Answer from the drawing. Dimensions are ordinates in mm from the lowest x, y and z of the part. A direction names the side the tool comes from. Coordinates: 2 decimals unless noted, no trailing zeros. Write each loop counter-clockwise with the first axis right and the second up, starting at its lowest first coordinate (ties: lowest second). Pieces come first, ordered by that corner, then holes. Notation, with made-up numbers: (26.25, 22) -> (41.25, 22) arc R32 cw to (41.25, 48) -> close; hole circle Ø2 at (56, 65). An arc over 180 degrees is marked (long way). Return JSON: item names as keys, results as strings.
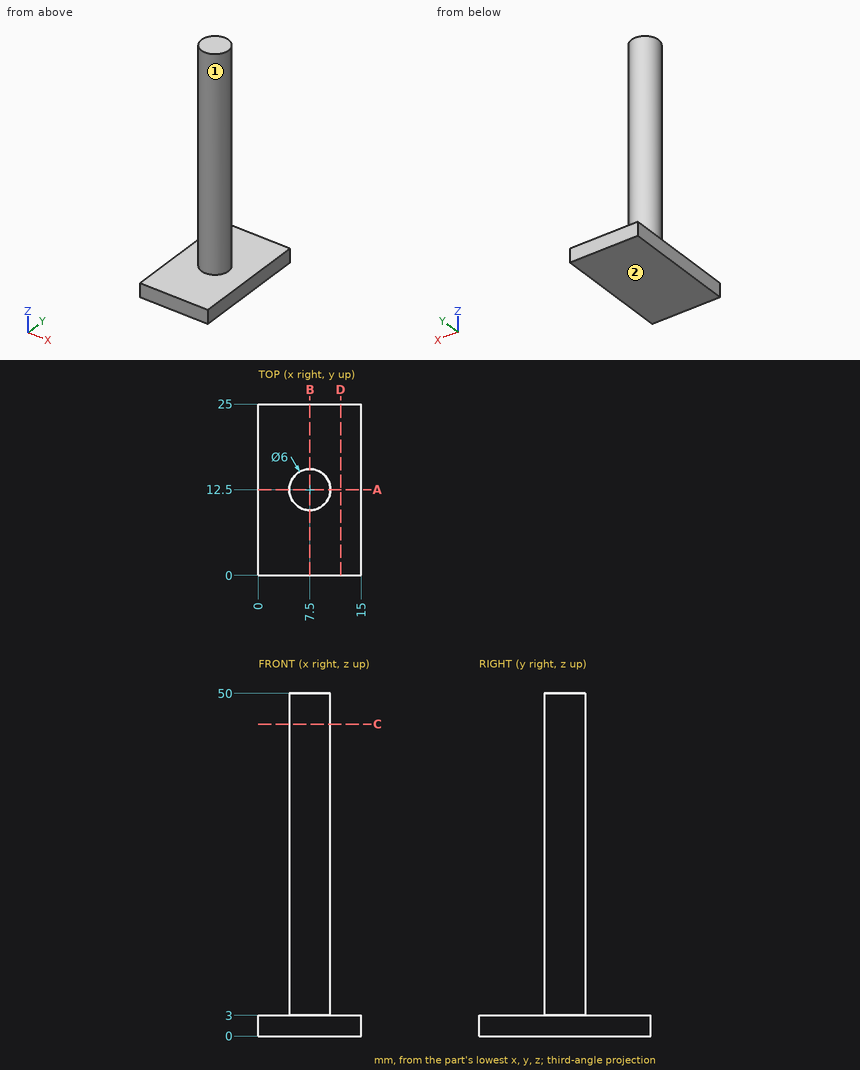
1. The part is cut by section D-D (x = 12). Determine the outline of the cut face in (y, z), then the cut area to 3 significant figures.
Taken from the geometry:
{"outline": "(0, 0) -> (25, 0) -> (25, 3) -> (0, 3) -> close", "area": "75.0 mm2"}
2. Flat-ended cylindrical pins translate along their axes: pin 1 Ø10 at (y, z) = (21, 36.5) entering from +X; pin 2 Ø7.5 at (x, y) = (7.5, 16.5) entering from +Z; pin 3 Ø6 at (x, z) = (4.5, 12) entering from -Y; pin 4 Ø1 at (x, z) = (10, 43) entering from -Y. Find the tip coordinate at first contact, or state that the pin passes through.
Taken from the geometry:
{"pin 1": "passes through", "pin 2": "stops at z = 50", "pin 3": "stops at y = 9.5", "pin 4": "stops at y = 10.26"}
3. The part is cut by section B-B (x = 7.5). Determine the outline of the cut face in (y, z).
Taken from the geometry:
{"outline": "(0, 0) -> (25, 0) -> (25, 3) -> (15.5, 3) -> (15.5, 50) -> (9.5, 50) -> (9.5, 3) -> (0, 3) -> close"}
4. A tool of negligible diameter and unlimited length cuts with its end or side. For the marked faces 1 and 2, from which of +Z, -Z, +X, -X, +Y, -Y can it reach the whole face along a straight path? Write none if from no direction.
Taken from the geometry:
{"face 1": "+Z", "face 2": "-Z, +X, -X, +Y, -Y"}
5. Consider L1, parallel to Z at x = 1.25, y = 14.75; L2, parallel to X at y = 12.5, z = 21.5; L3, parallel to X at y = 10.5, z = 21. Determine where each line is inside the solid, lowest interval first.
Taken from the geometry:
{"L1": "z = 0 to 3", "L2": "x = 4.5 to 10.5", "L3": "x = 5.26 to 9.74"}
6. The part is cut by section C-C (z = 45.5). Determine the outline of the cut face in (x, y), then the cut area to 3 significant figures.
Taken from the geometry:
{"outline": "circle Ø6 at (7.5, 12.5)", "area": "28.3 mm2"}
7. The part is cut by section A-A (y = 12.5). Determine the outline of the cut face in (x, z).
Taken from the geometry:
{"outline": "(0, 0) -> (15, 0) -> (15, 3) -> (10.5, 3) -> (10.5, 50) -> (4.5, 50) -> (4.5, 3) -> (0, 3) -> close"}
